Check sheet for the modelled part. Datum: model origin and axes. Units: mm. Face numbers are marked on the shaded views. A direction names the side the tool comes from. Round coordinates to 2 decimals unless told otherwise and drop trailing zeros. Loops run counter-clockwise (first coordinate to the right, second up) from the corner with the lowest first, then second, coordinate; pieces in that order, holes last. Notation, with made-up numbers: (31.5, 85) -> (51.5, 85) arc R16 cw to (51.5, 91) -> close; hole circle Ø2 at (0, 63.5). An arc over 180 degrees is marked (long way). Return JSON: item names as keys, results as strings.
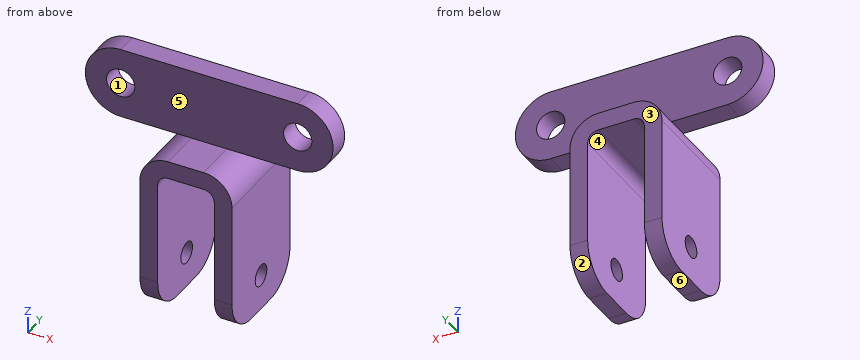
from build123d import *

# Parameters (mm, degrees)
EXTRUDE_THIN1_DEPTH     = 15
FILLET1_R               = 10
SKETCH2_R               = 4
BOSS_EXTRUDE1_DEPTH     = 3
CUT_EXTRUDE1_DEPTH      = 69.833131557
CUT_EXTRUDE1_DEPTH_BACK = 69.833131557


with BuildPart() as part:
    # Sketch1 → Extrude-Thin1 (new, symmetric)
    with BuildSketch(Plane(origin=(0, 0, 0), x_dir=(1, 0, 0), z_dir=(0, 1, 0))):
        with BuildLine():
            Line((-13, 47), (-13, 8))
            ThreePointArc((-13, 8), (-10.656854249, 2.343145751), (-5, 0))
            Line((-5, 0), (0, 0))
            Line((0, 0), (5, 0))
            ThreePointArc((5, 0), (10.656854249, 2.343145751), (13, 8))
            Line((13, 8), (13, 47))
            Line((13, 47), (8, 47))
            Line((8, 47), (8, 8))
            ThreePointArc((8, 8), (7.121320344, 5.878679656), (5, 5))
            Line((5, 5), (0, 5))
            Line((0, 5), (-5, 5))
            ThreePointArc((-5, 5), (-7.121320344, 5.878679656), (-8, 8))
            Line((-8, 8), (-8, 47))
            Line((-8, 47), (-13, 47))
        make_face()
    extrude(amount=EXTRUDE_THIN1_DEPTH, both=True)

    # Fillet1
    fillet1_edges = [part.edges().sort_by_distance(p)[0] for p in [
        (-10.5, -15, -47),
        (10.5, -15, -47),
        (-10.5, 15, -47),
        (10.5, 15, -47),
    ]]
    fillet(fillet1_edges, radius=FILLET1_R)

    # Sketch2 → Boss-Extrude1 (add, symmetric)
    with BuildSketch(Plane(origin=(0, 0, 0), x_dir=(1, 0, 0), z_dir=(0, 1, 0))):
        with BuildLine():
            Line((5, 0), (-5, 0))
            Line((-5, 0), (-25, 0))
            ThreePointArc((-25, 0), (-35, -10), (-25, -20))
            Line((-25, -20), (25, -20))
            ThreePointArc((25, -20), (35, -10), (25, 0))
            Line((25, 0), (5, 0))
        make_face()
        with Locations(Location((-25, -10, 0), (0, 0, 270))):
            Circle(SKETCH2_R, mode=Mode.SUBTRACT)
        with Locations(Location((25, -10, 0), (0, 0, 270))):
            Circle(SKETCH2_R, mode=Mode.SUBTRACT)
    extrude(amount=BOSS_EXTRUDE1_DEPTH, both=True)

    # Sketch3 → Cut-Extrude1 (cut, two sides: drawn at the far end of the back side and taken through both)
    with BuildSketch(Plane(origin=(13, 0, 0), x_dir=(0, 0, -1), z_dir=(1, 0, 0)).offset(-CUT_EXTRUDE1_DEPTH_BACK)):
        with BuildLine():
            ThreePointArc((40, 0), (37, 3), (34, 0))
            Line((34, 0), (40, 0))
        make_face()
        with BuildLine():
            Line((40, 0), (34, 0))
            ThreePointArc((34, 0), (37, -3), (40, 0))
        make_face()
    extrude(amount=CUT_EXTRUDE1_DEPTH + CUT_EXTRUDE1_DEPTH_BACK, mode=Mode.SUBTRACT)


solid = part.part
Q1. Section check D-D (z = 10). Record the boundary of the cut face in (x, y).
Results list:
{"outline": "(-35, -3) -> (-29, -3) -> (-29, 3) -> (-35, 3) -> close; (-21, -3) -> (21, -3) -> (21, 3) -> (-21, 3) -> close; (29, -3) -> (35, -3) -> (35, 3) -> (29, 3) -> close"}
Q2. Material ranges on line 1 (X direction, y = 0.7, z = 10); line 2 (Y direction, x = -10.75, z = -37); line 3 (X direction, y = 3.5, z = -12), recorded low to high.
Results list:
{"line 1": "-35 to -29, -21 to 21, 29 to 35", "line 2": "-15 to -3, 3 to 15", "line 3": "-13 to -8, 8 to 13"}
Q3. Section check B-B (z = -10). Record the boundary of the cut face in (x, y).
Results list:
{"outline": "(-13, -15) -> (-8, -15) -> (-8, 15) -> (-13, 15) -> close; (8, -15) -> (13, -15) -> (13, 15) -> (8, 15) -> close"}
Q4. Section check A-A (y = 0). Record the boundary of the cut face in (x, z).
Results list:
{"outline": "(-25, 0) -> (-5, 0) arc R8 ccw to (-13, -8) -> (-13, -34) -> (-8, -34) -> (-8, -8) arc R3 cw to (-5, -5) -> (5, -5) arc R3 cw to (8, -8) -> (8, -34) -> (13, -34) -> (13, -8) arc R8 ccw to (5, 0) -> (25, 0) arc R10 ccw to (25, 20) -> (-25, 20) arc R10 ccw to start; (-13, -47) -> (-8, -47) -> (-8, -40) -> (-13, -40) -> close; (8, -47) -> (13, -47) -> (13, -40) -> (8, -40) -> close; hole circle Ø8 at (-25, 10); hole circle Ø8 at (25, 10)"}
Q5. Draft check along Z on the marked faces 1, 2 and 3. Enter one of: released by +Z, released by -Z, zero draft, split by the parting line, or undercut.
Results list:
{"face 1": "undercut", "face 2": "released by -Z", "face 3": "zero draft"}
Q6. Section check C-C (x = -27.5). Record the boundary of the cut face in (y, z).
Results list:
{"outline": "(-3, 0.32) -> (3, 0.32) -> (3, 6.88) -> (-3, 6.88) -> close; (-3, 13.12) -> (3, 13.12) -> (3, 19.68) -> (-3, 19.68) -> close"}
Q7. Tool access check on the marked faces 4, 5 and 6. Record the directions out of +Z, -Z, +X, -X, +Y, -Y that give a thin tool (end or side, any length) a straight path to the whole face; none if there is none.
Results list:
{"face 4": "-Z, +Y, -Y", "face 5": "+Z, +X, -X, -Y", "face 6": "-Z, +X, -X, +Y, -Y"}
Q8. Go/stop test with flat-tipped pins: pin 1 (9 mm diameter, centred on x = -25, z = 10, fed in from -Y); pin 2 (11 mm diameter, centred on x = -1.5, y = 9, fed in from +Z); pin 3 (9 mm diameter, centred on y = -2.5, z = -20, fed in from +X); pin 4 (10 mm diameter, centred on x = -15, z = -5.5, fed in from -Y). Record where each tip stops, or that it passes through.
Results list:
{"pin 1": "y = -3", "pin 2": "z = 0", "pin 3": "x = 13", "pin 4": "y = -15"}
